Read the model definition and answer for the solid it produces. Units are mm, in the model's axes. A direction names the side the tool comes from. Round coordinates to 2 decimals unless told otherwise and drop trailing zeros. Answer as CSV lines item,"result".
```python
from build123d import *

# Parameters (mm, degrees)
F3_DEPTH = 15


with BuildPart() as f1:
    # F0 (on Front) → F1 (revolve)
    with BuildSketch(Plane.XZ):
        Polygon((-24, 3.25), (-49, 3.25), (-49, 0), (40, 0), (40, 12), (0, 12), (0, 3.4), (-2, 3.4), (-2, 8), (-24, 8), align=None)
    revolve(axis=Axis((-4.5, 0, 0), (-1, 0, 0)))


with BuildPart() as f3:
    # F2 (on Front) → F3 (new body)
    with BuildSketch(Plane.XZ):
        with BuildLine():
            add(Edge.make_bspline(
                [(-49.041996, 5), (-24.702918, 11.935834), (-28.770125, 17), (42.303421, 15)],
                knots=[0, 0, 0, 0, 91.891159, 91.891159, 91.891159, 91.891159], degree=3))
            Line((-49.041996, 5), (-49.041996, -5))
            add(Edge.make_bspline(
                [(-49.041996, -5), (-24.702918, -11.935834), (-28.770125, -17), (42.303421, -15)],
                knots=[0, 0, 0, 0, 91.891159, 91.891159, 91.891159, 91.891159], degree=3))
            add(Edge.make_bspline(
                [(42.303421, 15), (51.051009, 14.836123), (64.952584, -0.003986), (51.450081, -14.828151), (42.303421, -15)],
                knots=[0, 0, 0, 0, 21.784888, 43.569776, 43.569776, 43.569776, 43.569776], degree=3))
        make_face()
    extrude(amount=F3_DEPTH)

    # F4: cut F1
    add(f1.part, mode=Mode.SUBTRACT)


solid = f3.part
```
1) Determine the mould class of faces 1 (the flat face through (0, -6, 0)), 2 (the flat face through (-0.2, 0, -3.7)) for opening direction Z: released by +Z, released by -Z, zero draft, split by the parting line, or undercut.
Evaluation:
face 1,"undercut"
face 2,"zero draft"
2) Each of these flat-tipped pins is pushed along its axis until it touches: P1, Ø4, axis at x = 45, y = -13, coming from the -Z side; P2, Ø5, axis at x = -12, y = -8, coming from the -Z side; P3, Ø4, axis at y = -4.5, z = -2.5, coming from the +X side. Where does it stop, or does it pass through?
Evaluation:
P1,"stops at z = -14.97"
P2,"stops at z = -14.7"
P3,"stops at x = 58.1"
3) A tool of negligible diameter and unlimited length cuts with its end or side. For faces 3 (the cylindrical face through (-36.67, -3.25, -0.07)), 4 (the flat face through (9, -15, 0)), from which of +Z, -Z, +X, -X, +Y, -Y can it reach the whole face along a straight path? Write none if from no direction.
Evaluation:
face 3,"+Y"
face 4,"+Z, -Z, +X, -X, -Y"
4) Straight lines are drawn through the part: line 1 (X direction, y = -6.25, z = -4.5); line 2 (Z direction, x = -14.5, y = -2.25); line 3 (X direction, y = -7, z = -1). For each, find the intervals that lie inside material, in ascending order.
Evaluation:
line 1,"x = -49.04 to -24, -2 to 0, 40 to 57.34"
line 2,"z = -14.24 to -7.68, 7.68 to 14.24"
line 3,"x = -49.04 to -24, -2 to 0, 40 to 58.07"
5) Find section A-A, the plane y = -7. Count the separate pieces of the cut face and the enclosed holes in it, then the cut area to 3 significant figures.
Evaluation:
separate pieces,"1"
enclosed holes,"2"
area,"1,850 mm^2"
